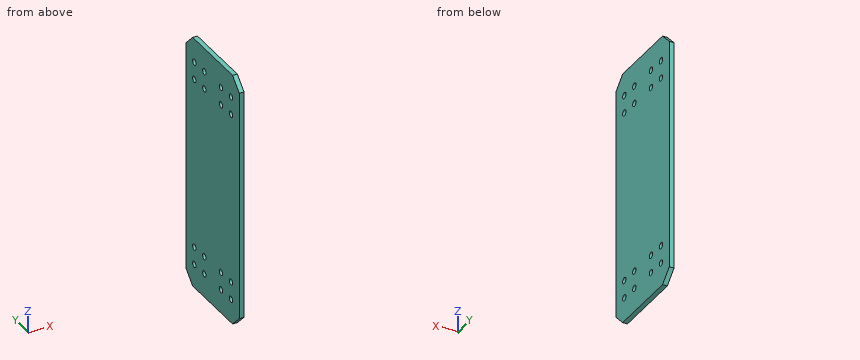
Autodesk Inventor part; units mm, degrees
ref_plane "YZ Plane" through (0, 0, 0) normal (1, 0, 0) x (0, 1, 0)
ref_plane "XZ Plane" through (0, 0, 0) normal (0, 1, 0) x (-1, 0, 0)
ref_plane "XY Plane" through (0, 0, 0) normal (0, 0, 1) x (1, 0, 0)
sketch "Sketch1" plane through (0, 0, 0) normal (1, 0, 0) x (0, 1, 0)
  line L0 (-32, 86) -> (32, 86)
  line L1 (32, 86) -> (32, -86)
  line L2 (32, -86) -> (-32, -86)
  line L3 (-32, -86) -> (-32, 86)
  line L4 (-32, 86) -> (32, -86) construction
  line L5 (32, 86) -> (-32, -86) construction
  point P0 (0, 0)
  dimension "d0" = 64
  dimension "d1" = 172
extrude "Extrusion1" add sketch "Sketch1" along normal blind 3.175
sketch "Sketch2" plane through (3.175, 0, 0) normal (1, 0, 0) x (0, 0, -1)
  circle A0 centre (-64, -16) radius 2.5 construction
  circle A1 centre (-70, -22) radius 2
  circle A2 centre (-58, -22) radius 2
  circle A3 centre (-58, -10) radius 2
  circle A4 centre (-70, -10) radius 2
  line L0 (-86, 32) -> (-86, -32) construction
  line L1 (-86, 0) -> (86, 0) construction
  line L2 (86, -32) -> (86, 32) construction
  line L3 (86, 32) -> (-86, 32) construction
  line L4 (0, 32) -> (0, -32) construction
  line L5 (-86, -32) -> (86, -32) construction
  circle A5 centre (-64, 16) radius 2.5 construction
  circle A6 centre (-70, 22) radius 2
  circle A7 centre (-58, 22) radius 2
  circle A8 centre (-58, 10) radius 2
  circle A9 centre (-70, 10) radius 2
  circle A10 centre (64, -16) radius 2.5 construction
  circle A11 centre (70, -22) radius 2
  circle A12 centre (58, -22) radius 2
  circle A13 centre (58, -10) radius 2
  circle A14 centre (70, -10) radius 2
  circle A15 centre (64, 16) radius 2.5 construction
  circle A16 centre (70, 22) radius 2
  circle A17 centre (58, 22) radius 2
  circle A18 centre (58, 10) radius 2
  circle A19 centre (70, 10) radius 2
  point P0 (0, 0)
  dimension "d4" = 5
  dimension "d5" = 64
  dimension "d6" = 16
  dimension "d7" = 4
  dimension "d8" = 6
  dimension "d9" = 6
  dimension "d12" = 360
chamfer "Chamfer1" distance 8 angle 45 4 edges at (1.5875, 32, 86) (1.5875, -32, 86) (1.5875, -32, -86) (1.5875, 32, -86)
extrude "Extrusion2" cut sketch "Sketch2" against normal through all
properties part number "ArmBaseSupportPlates"
Check sheet for the modelled part. Datum: model origin and axes. Units: mm. Give positions to 0.01 mm unless a question says otherwise; leave off trailing zeros. Loops run counter-clockwise (first coordinate to the right, second up) from the corner with the lowest first, then second, coordinate; pieces in that order, holes last. Notation, with made-up numbers: M 27.25,73 L 46.25,73 A6 cw 46.25,81 Z; hole C 2.25,-10.75 d3. An arc over 180 degrees is marked long. Answer in a Markdown table with one row per item.
1) Cross-section at B-B (y = 22). Enter the section's corners in (x, z) (3 decimals).
Solutions:
| item | result |
|---|---|
| outline | M 0,-86 L 3.175,-86 L 3.175,-72 L 0,-72 Z; M 0,-68 L 3.175,-68 L 3.175,-60 L 0,-60 Z; M 0,-56 L 3.175,-56 L 3.175,56 L 0,56 Z; M 0,60 L 3.175,60 L 3.175,68 L 0,68 Z; M 0,72 L 3.175,72 L 3.175,86 L 0,86 Z |
2) Thickness scan on line 1 (Y direction, x = 2.45, z = -70); line 2 (Z direction, x = 2.25, y = 29). Record the ranges inside material, lowest first.
Solutions:
| item | result |
|---|---|
| line 1 | y = -32 to -24, -20 to -12, -8 to 8, 12 to 20, 24 to 32 |
| line 2 | z = -81 to 81 |
3) Cross-section at A-A (z = 58). Enter the section's corners in (x, y) (3 decimals), plus the area to 3 significant figures.
Solutions:
| item | result |
|---|---|
| outline | M 0,-32 L 3.175,-32 L 3.175,-24 L 0,-24 Z; M 0,-20 L 3.175,-20 L 3.175,-12 L 0,-12 Z; M 0,-8 L 3.175,-8 L 3.175,8 L 0,8 Z; M 0,12 L 3.175,12 L 3.175,20 L 0,20 Z; M 0,24 L 3.175,24 L 3.175,32 L 0,32 Z |
| area | 152 mm^2 |
4) Cross-section at C-C (x = 1). Count the separate pieces of the cut face and the enclosed holes in it, plus the area to 3 significant figures.
Solutions:
| item | result |
|---|---|
| separate pieces | 1 |
| enclosed holes | 16 |
| area | 10,700 mm^2 |
